Autodesk Inventor part; units mm, degrees
ref_plane "YZ Plane" through (0, 0, 0) normal (1, 0, 0) x (0, 1, 0)
ref_plane "XZ Plane" through (0, 0, 0) normal (0, 1, 0) x (-1, 0, 0)
ref_plane "XY Plane" through (0, 0, 0) normal (0, 0, 1) x (1, 0, 0)
sketch "Sketch1" plane through (0, 0, 0) normal (0, 1, 0) x (-1, 0, 0)
  line L0 (0, 0) -> (-38.1, 0)
  line L1 (-38.1, 0) -> (-38.1, -88.9)
  line L2 (-38.1, -88.9) -> (0, -88.9)
  line L3 (0, -88.9) -> (0, 0)
  dimension "d0" = 38.1
  dimension "d1" = 88.9
extrude "Extrusion1" add sketch "Sketch1" along normal blind 355.6
sketch "Sketch3" plane through (0, 355.6, 0) normal (0, 1, 0) x (1, 0, 0)
  line L0 (0, 88.9) -> (0, 0)
  line L1 (0, 74.725) -> (18.45, 74.725)
  line L2 (18.45, 74.725) -> (18.45, 0) construction
  line L3 (18.45, 0) -> (0, 0)
  line L4 (0, 0) -> (0, 74.725)
  line L5 (38.1, 88.9) -> (0, 88.9)
  line L6 (18.45, 74.725) -> (18.45, 61.2)
  line L7 (18.45, 74.725) -> (18.45, 14.175)
  line L8 (18.45, 44.45) -> (24.45, 44.45)
  line L9 (0, 0) -> (38.1, 0)
  dimension "d35" = 60.55
  dimension "d42" = 6
  dimension "d43" = 30.275
  dimension "d45" = 14.175
  dimension "d46" = 14.175
  dimension "d48" = 24.45
  dimension "d49" = 44.45
hole "Hole1" at (18.45, 355.6, -74.725) at (24.45, 355.6, -44.45) at (18.45, 355.6, -14.175) direction (0, -1, 0) diameter 7 depth 10 tip angle 118
sketch "Sketch4" plane through (38.1, 0, 0) normal (1, 0, 0) x (0, 0, -1)
  line L0 (0, 0) -> (88.9, 0)
  line L1 (0, 0) -> (44.45, 0) construction
  line L2 (44.45, 0) -> (44.45, 20) construction
  line L3 (44.45, 20) -> (0, 20) construction
  line L4 (0, 20) -> (0, 0) construction
  dimension "d25" = 44.45
  dimension "d26" = 20
hole "Hole2" at (38.1, 20, -44.45) direction (-1, 0, 0) diameter 6.5 depth 10
properties part number "shin2x4" material "Wood (Birch)"
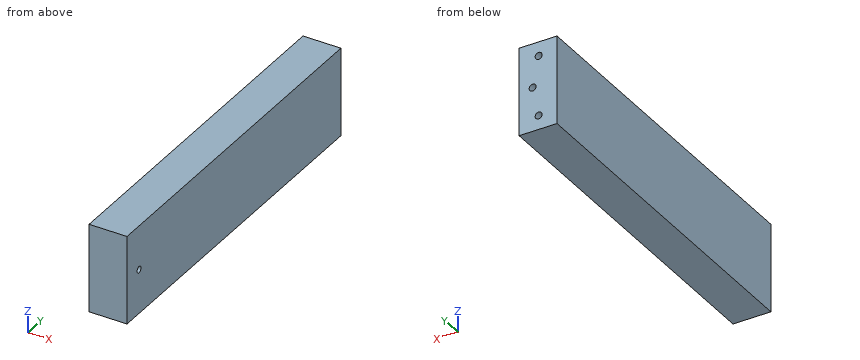
For this review, take the finished solid that the model builds, in its own axes (mm). Coordinates: 2 decimals unless noted, no trailing zeros. Write each loop counter-clockwise with the first axis right and the second up, starting at its lowest first coordinate (ties: lowest second). Pieces come first, ordered by that corner, then holes. Notation, with made-up numbers: (54, -22.5) - (84, -22.5) arc R13 ccw to (84, 1.5) - close; hole circle Ø5 at (45, 50.5). An arc over 180 degrees is marked (long way). Answer in a Markdown table with one row per item. Add a question column.
Q1. For probe 1 along X at (y, z) = (348, -44); probe 2 along Z at (x, y) = (33, 20); probe 3 along Y at (x, z) = (20.5, -74), list the stretches that pass through material, from the lowest coordinate up.
Q2. For P1, Ø6, axis at y = 20, z = -44.45, coming from the -X side, flat-tipped, find the tip position at first contact; note if it passes through.
Q3. We need section A-A, the plane y = 20. State the section outline as (x, z) points, and give its area (3 significant figures).
Answer list:
| question | item | result |
|---|---|---|
| 1 | probe 1 | x = 0 to 20.98, 27.92 to 38.1 |
| 1 | probe 2 | z = -88.9 to -47.7, -41.2 to 0 |
| 1 | probe 3 | y = 0 to 344.8 |
| 2 | P1 | stops at x = 0 |
| 3 | outline | (0, -88.9) - (38.1, -88.9) - (38.1, -47.7) - (28.1, -47.7) - (28.1, -41.2) - (38.1, -41.2) - (38.1, 0) - (0, 0) - close |
| 3 | area | 3,320 mm2 |
